Part model, mm, in its own coordinate system. A direction names the side the tool comes from. Give positions to 0.01 mm unless a question says otherwise; leave off trailing zeros. Order: outer loops, then holes, each group sorted by start corner. A loop starts at its lowest first (then second) coordinate and runs counter-clockwise, first axis right, second up. Notation, with made-up numbers: (-7, 83) -> (2, 83) arc R20 ccw to (2, 89) -> close; hole circle Ø4 at (-24, -12.75). An arc over 180 degrees is marked (long way). Write item = value, one per line. Start each with the question number.
Item 1: Tool access for faces 4 (the face through (16.98, 15.62, -3.47)), 5 (the face through (37, 25, 0)): list every direction of +Z, -Z, +X, -X, +Y, -Y with a clear straight run to the whole face (end or side of a thin tool).
Item 2: Band-saw the part on A-A on z = 0. Write the cut outline in (x, y).
Item 3: Pull direction Y, two halves, no side cores. Call faces 1 (the face through (37, -20, 0)), 2 (the face through (36.635, 34.168, -7.587)), 3 (the face through (14.45, 15, 7)): +Y half, -Y half, draft (parallel to the pull), parting line (faces both ways), or undercut.
Item 4: Band-saw the part on C-C on x = 53. Write the cut outline in (y, z), plus the area to 3 significant figures.
Item 5: Band-saw the part on B-B on y = 22.5. Write the cut outline in (x, z), plus the area to 3 significant figures.
Item 6: Flat gauge pins, fed straight in: P1, Ø4, axis at y = 11.25, z = -19.49, coming from the +X side; P2, Ø2, axis at x = 33.5, y = 8.5, coming from the -Z side; P3, Ø2, axis at x = 45, y = 23, coming from the +Z side; P4, Ø4, axis at x = 19.5, z = -18, coming from the -Y side. Where does each tip first touch, or does it go through?
Item 7: Band-saw the part on D-D on y = -11.25. Write the cut outline in (x, z), plus the area to 3 significant figures.
Item 8: Drill centre lines: line 1 along Y through (x, z) = (45, 0); line 2 along Y through (x, z) = (21.5, 20); line 3 along Y through (x, z) = (20.5, -18.5). Where is each one in solid material? Low to high.
```python
from build123d import *

# Parameters (mm, degrees)
SKETCH2_R          = 2.5
CUT_EXTRUDE1_DEPTH = 45


with BuildPart() as part:
    # Sketch1 → Revolve1 (revolve)
    with BuildSketch(Plane.XY, mode=Mode.PRIVATE) as revolve1_sk:
        Polygon((14.45, 35), (14.45, 16), (19.45, 16), (19.45, 5), (59.45, 5), (59.45, 35), align=None)
    revolve(revolve1_sk.sketch.rotate(Axis((0, 0, 0), (1, 0, 0)), 90), axis=Axis((0, 0, 0), (1, 0, 0)))

    # Sketch2 → Cut-Extrude1 (cut)
    with BuildSketch(Plane.ZY.offset(-14.45)):
        with Locations((19.485571585, 11.25)):
            Circle(SKETCH2_R)
        with Locations((19.485571585, -11.25)):
            Circle(SKETCH2_R)
        with Locations((0, -22.5)):
            Circle(SKETCH2_R)
        with Locations((-19.485571585, -11.25)):
            Circle(SKETCH2_R)
        with Locations((-19.485571585, 11.25)):
            Circle(SKETCH2_R)
        with Locations((0, 22.5)):
            Circle(SKETCH2_R)
    extrude(amount=-CUT_EXTRUDE1_DEPTH, mode=Mode.SUBTRACT)


solid = part.part
```
Values found:
q1.face_4 = -X
q1.face_5 = +X, -X
q2.outline = (14.45, -35) -> (59.45, -35) -> (59.45, -25) -> (14.45, -25) -> close; (14.45, -20) -> (59.45, -20) -> (59.45, -5) -> (19.45, -5) -> (19.45, -16) -> (14.45, -16) -> close; (14.45, 16) -> (19.45, 16) -> (19.45, 5) -> (59.45, 5) -> (59.45, 20) -> (14.45, 20) -> close; (14.45, 25) -> (59.45, 25) -> (59.45, 35) -> (14.45, 35) -> close
q3.face_1 = undercut
q3.face_2 = parting line
q3.face_3 = draft
q4.outline = circle Ø70 at (0, 0); hole circle Ø5 at (-22.5, 0); hole circle Ø5 at (-11.25, -19.49); hole circle Ø5 at (-11.25, 19.49); hole circle Ø10 at (0, 0); hole circle Ø5 at (11.25, -19.49); hole circle Ø5 at (11.25, 19.49); hole circle Ø5 at (22.5, 0)
q4.area = 3,650 mm^2
q5.outline = (14.45, -26.81) -> (59.45, -26.81) -> (59.45, -2.5) -> (14.45, -2.5) -> close; (14.45, 2.5) -> (59.45, 2.5) -> (59.45, 26.81) -> (14.45, 26.81) -> close
q5.area = 2,190 mm^2
q6.P1 = through
q6.P2 = -34.19
q6.P3 = 27.22
q6.P4 = -31.13
q7.outline = (14.45, -33.14) -> (59.45, -33.14) -> (59.45, -21.99) -> (14.45, -21.99) -> close; (14.45, -16.99) -> (59.45, -16.99) -> (59.45, 16.99) -> (14.45, 16.99) -> (14.45, 11.38) -> (19.45, 11.38) -> (19.45, -11.38) -> (14.45, -11.38) -> close; (14.45, 21.99) -> (59.45, 21.99) -> (59.45, 33.14) -> (14.45, 33.14) -> close
q7.area = 2,420 mm^2
q8.line_1 = -35 to -25, -20 to -5, 5 to 20, 25 to 35
q8.line_2 = -28.72 to -13.7, -8.8 to 8.8, 13.7 to 28.72
q8.line_3 = -29.71 to -13.55, -8.95 to 8.95, 13.55 to 29.71
